from build123d import *

# Parameters (mm, degrees)
SKETCH1_R           = 1.5
SHAPE_DEPTH         = 2.5
CHAMFER_2_SIZE      = 0.2
SKETCH2_R           = 2.55
SKETCH2_R_2         = 1.5
BOSS_EXTRUDE2_DEPTH = 1.5
FILLET1_R           = 0.2
CUT_EXTRUDE1_START  = -0.1
SKETCH3_R           = 2.35
SKETCH3_R_2         = 1.5
CUT_EXTRUDE1_DEPTH  = 0.1


with BuildPart() as part:
    # Sketch1 → Shape (new body)
    with BuildSketch(Plane.XY):
        Polygon((-1.58771324, -2.75), (1.58771324, -2.75), (3.175426481, 0), (1.58771324, 2.75), (-1.58771324, 2.75), (-3.175426481, 0), align=None)
        Circle(SKETCH1_R, mode=Mode.SUBTRACT)
    extrude(amount=SHAPE_DEPTH)

    # Chamfer 2
    chamfer_2_edges = [part.edges().sort_by_distance(p)[0] for p in [
        (2.38156986, -1.375, 2.5),
        (2.38156986, 1.375, 2.5),
        (0, 2.75, 2.5),
        (-2.38156986, 1.375, 2.5),
        (-2.38156986, -1.375, 2.5),
        (-2.38156986, 1.375, 0),
        (0, 2.75, 0),
        (2.38156986, 1.375, 0),
        (0, -2.75, 2.5),
        (2.38156986, -1.375, 0),
        (0, -2.75, 0),
        (-2.38156986, -1.375, 0),
    ]]
    chamfer(chamfer_2_edges, length=CHAMFER_2_SIZE)

    # Sketch2 → Boss-Extrude2 (add)
    with BuildSketch(Plane.XY.offset(2.5)):
        with Locations(Location((0, 0, 0), (0, 0, 150))):
            Circle(SKETCH2_R)
        Circle(SKETCH2_R_2, mode=Mode.SUBTRACT)
    extrude(amount=BOSS_EXTRUDE2_DEPTH)

    # Fillet1
    fillet1_edges = [part.edges().sort_by_distance(p)[0] for p in [
        (2.20836478, -1.275, 4),
    ]]
    fillet(fillet1_edges, radius=FILLET1_R)

    # Sketch3 → Cut-Extrude1 (cut)
    with BuildSketch(Plane.XY.offset(4).offset(CUT_EXTRUDE1_START)):
        Circle(SKETCH3_R)
        Circle(SKETCH3_R_2, mode=Mode.SUBTRACT)
    extrude(amount=CUT_EXTRUDE1_DEPTH, mode=Mode.SUBTRACT)


solid = part.part
Geometry check sheet. Reference: the model listing, model coordinates, mm. A direction names the side the tool comes from. Round coordinates to 2 decimals unless told otherwise and drop trailing zeros. Order: outer loops, then holes, each group sorted by start corner. A loop starts at its lowest first (then second) coordinate and runs counter-clockwise, first axis right, second up. Notation, with made-up numbers: M 45.5,-28.5 L 85.5,-28.5 A26 cw 85.5,4.5 Z; hole C 73.25,39.5 d2. An arc over 180 degrees is marked long. Answer in a Markdown table with one row per item. Add a question column.
Item 1: Sectioned sample at B-B, the plane z = 3.45. Enter the section's corners in (x, y) (3 decimals), plus the area to 3 significant figures.
Item 2: Depth check by flat-ended pin: pin 1 Ø2 at (y, z) = (2, 3) entering from +X; pin 2 Ø1.4 at (x, y) = (1, -1) entering from +Z. Enter the tip coordinate at first touch or a pass-through.
Item 3: Material ranges on L1, parallel to Y at x = 0, z = 2.75; L2, parallel to Y at x = 0, z = 1.3; L3, parallel to Z at x = -1.5, y = -1.4, recorded low to high. Write a range as [from, to].
Item 4: Draft check along X on faces 3 (the face through (-1.5, 0.07, 1.92)), 4 (the face through (0, -2.75, 1)), 5 (the face through (2.37, -1.394, 1.235)). Enter one of: released by +X, released by -X, zero draft, split by the parting line, or undercut.
Item 5: Sectioned sample at A-A, the plane z = 0.45. Enter the section's corners in (x, y).
Item 6: Set-up check for faces 1 (the face through (0, -2, 3.9)), 2 (the face through (1.3, -1.1, 0)): record each of +Z, -Z, +X, -X, +Y, -Y from which the full face is reachable in a straight line by a thin tool's end or side.
Filled in:
| question | item | result |
|---|---|---|
| 1 | outline | C 0,0 d5.1; hole C 0,0 d3 |
| 1 | area | 13.4 mm² |
| 2 | pin 1 | stops at x = 2.43 |
| 2 | pin 2 | stops at z = 3.9 |
| 3 | L1 | y = [-2.55, -1.5], [1.5, 2.55] |
| 3 | L2 | y = [-2.75, -1.5], [1.5, 2.75] |
| 3 | L3 | z = [0, 3.9] |
| 4 | face 3 | undercut |
| 4 | face 4 | zero draft |
| 4 | face 5 | released by +X |
| 5 | outline | M -3.18,0 L -1.59,-2.75 L 1.59,-2.75 L 3.18,0 L 1.59,2.75 L -1.59,2.75 Z; hole C 0,0 d3 |
| 6 | face 1 | +Z |
| 6 | face 2 | -Z, +X, -X, +Y, -Y |
